from build123d import *

# Parameters (mm, degrees)
SKETCH5_W           = 10
SKETCH5_H           = 5
BOSS_EXTRUDE2_DEPTH = 5


with BuildPart() as part:
    # Sketch5 → Boss-Extrude2 (new body)
    with BuildSketch(Plane.XY):
        Polygon((-16, -70), (16, -70), (16, -30), (95.875, -30), (95.875, 30), (16, 30), (16, 70), (-16, 70), (-16, 30), (-95.875, 30), (-95.875, -30), (-16, -30), align=None)
        with Locations((60, -25)):
            Rectangle(SKETCH5_W, SKETCH5_H, mode=Mode.SUBTRACT)
        with Locations((60, 25)):
            Rectangle(SKETCH5_W, SKETCH5_H, mode=Mode.SUBTRACT)
        with Locations((0, -25)):
            Rectangle(SKETCH5_W, SKETCH5_H, mode=Mode.SUBTRACT)
        with Locations((0, 25)):
            Rectangle(SKETCH5_W, SKETCH5_H, mode=Mode.SUBTRACT)
        with Locations((-60, 25)):
            Rectangle(SKETCH5_W, SKETCH5_H, mode=Mode.SUBTRACT)
        with Locations((-60, -25)):
            Rectangle(SKETCH5_W, SKETCH5_H, mode=Mode.SUBTRACT)
        with BuildLine():
            Line((6, 55), (6, 40))
            ThreePointArc((6, 40), (0, 34), (-6, 40))
            Line((-6, 40), (-6, 55))
            ThreePointArc((-6, 55), (0, 61), (6, 55))
        make_face(mode=Mode.SUBTRACT)
        with BuildLine():
            Line((-6, -40), (-6, -55))
            ThreePointArc((-6, -55), (0, -61), (6, -55))
            Line((6, -55), (6, -40))
            ThreePointArc((6, -40), (0, -34), (-6, -40))
        make_face(mode=Mode.SUBTRACT)
    extrude(amount=BOSS_EXTRUDE2_DEPTH)


solid = part.part
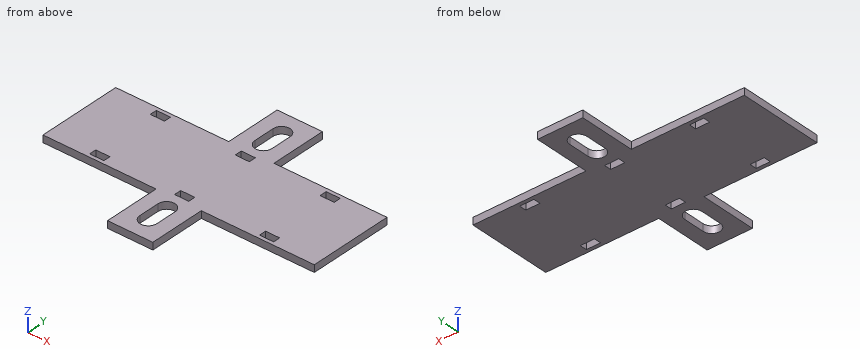
Design review of the part built by this model. Coordinates are the model's own, in mm. Round coordinates to 2 decimals unless told otherwise and drop trailing zeros. Loops run counter-clockwise (first coordinate to the right, second up) from the corner with the lowest first, then second, coordinate; pieces in that order, holes last. Notation, with made-up numbers: (18, 54) -> (62, 54) arc R23 cw to (62, 69) -> close; hole circle Ø8 at (80.25, 84). An arc over 180 degrees is marked (long way). Use one line per item in the form item = value. Start each with the question number.
Q1. We need section C-C on z = 3.4. State how many separate pieces and enclosed holes the cut face has, then the cut area to 3 significant figures.
Q2. We need section B-B on x = 0. Give the boundary of the cut face in (y, z).
Q3. Wall thickness on line 1 along X through (y, z) = (-54.5, 3); line 2 along Y through (x, z) = (-18, 2.8); line 3 along X through (y, z) = (-64, 3.3): over which ranges is each line inside the solid? List them lowest first. Write a range as [from, to].
Q4. We need section D-D on x = -28. Give the boundary of the cut face in (y, z), then the cut area to 3 significant figures.
Q5. We need section A-A on y = 48. Give the boundary of the cut face in (x, z), then the cut area to 3 significant figures.
Q6. For pin 1 Ø1.5 at (y, z) = (55, 2.5) entering from +X, flat-tipped, find the tip position at first contact; note if it passes through.
Calculated:
q1.separate_pieces = 1
q1.enclosed_holes = 8
q1.area = 13,200 mm²
q2.outline = (-70, 0) -> (-61, 0) -> (-61, 5) -> (-70, 5) -> close; (-34, 0) -> (-27.5, 0) -> (-27.5, 5) -> (-34, 5) -> close; (-22.5, 0) -> (22.5, 0) -> (22.5, 5) -> (-22.5, 5) -> close; (27.5, 0) -> (34, 0) -> (34, 5) -> (27.5, 5) -> close; (61, 0) -> (70, 0) -> (70, 5) -> (61, 5) -> close
q3.line_1 = [-16, -6], [6, 16]
q3.line_2 = [-30, 30]
q3.line_3 = [-16, 16]
q4.outline = (-30, 0) -> (30, 0) -> (30, 5) -> (-30, 5) -> close
q4.area = 300 mm²
q5.outline = (-16, 0) -> (-6, 0) -> (-6, 5) -> (-16, 5) -> close; (6, 0) -> (16, 0) -> (16, 5) -> (6, 5) -> close
q5.area = 100 mm²
q6.pin_1 = 16
